Read the model definition and answer for the solid it produces. Units are mm, in the model's axes. Face numbers are marked on the shaded views. Coordinates: 2 decimals unless noted, no trailing zeros. Loops run counter-clockwise (first coordinate to the right, second up) from the corner with the lowest first, then second, coordinate; pieces in that order, holes last. Notation, with made-up numbers: M -37,28 L -19,28 A27 ccw -19,66 Z; hole C -21.75,6.25 d3. An arc over 180 degrees is marked long. One line per item, written item: value. Start each with the question number.
1. The part is cut by section B-B (z = 19). Write down the section's boundary in (x, y).
2. The part is cut by section A-A (x = 18.5). Write down the section's boundary in (y, z).
3. Determine the mould class of the marked faces 1, 2, 3 and 4 for opening direction Z: +Z half, -Z half, draft (parallel to the pull), parting line (faces both ways), or undercut.
4. Consider probe 1 along Y at (x, z) = (3, 30); probe 2 along Z at (x, y) = (27.5, -49.5); probe 3 along Y at (x, z) = (17.25, 27.5). Determine where each line is inside the solid, lowest interval first.
5. Flat-ended cylindrical pins translate along their axes: pin 1 (5 mm diameter, centred on x = 18.5, y = -61.5, fed in from +Z); pin 2 (8 mm diameter, centred on x = 8, y = -47.5, fed in from +Z); pin 3 (12 mm diameter, centred on x = 12, z = 41, fed in from -Y). Find the tip coordinate at first contact, or state that the pin passes through.
6. The part is cut by section C-C (y = -58). Write down the section's boundary in (x, z), then the cut area to 3 significant figures.
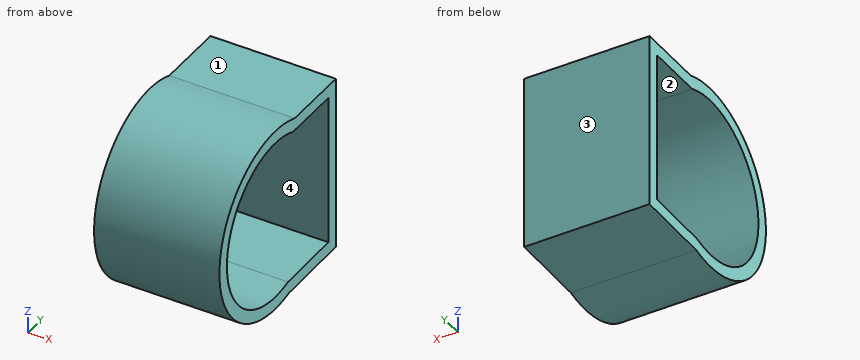
```python
from build123d import *

# Parameters (mm, degrees)
F1_DEPTH = 30
F2_T     = 3


with BuildPart() as f1:
    # F0 (on Right) → F1 (new body)
    with BuildSketch(Plane.YZ):
        with BuildLine():
            ThreePointArc((-50.5638438315, 48.3802992553), (-77.1344876234, 31.6163385121), (-52.6412177761, 11.9412470637))
            Line((-52.6412177761, 11.9412470637), (-36.4591793272, 12.1873354573))
            Line((-36.4591793272, 12.1873354573), (-36.4591793272, 42.854900606))
            Line((-36.4591793272, 42.854900606), (-36.4591793272, 48.3802992553))
            Line((-36.4591793272, 48.3802992553), (-38.9720265736, 48.3802992553))
            Line((-38.9720265736, 48.3802992553), (-50.5638438315, 48.3802992553))
        make_face()
    extrude(amount=F1_DEPTH)

    # F2
    f2_openings = [f1.faces().sort_by_distance(p)[0] for p in [
        (30, -55.280278, 30.40174),
        (0, -55.280278, 30.40174),
    ]]
    offset(amount=F2_T, openings=f2_openings, kind=Kind.INTERSECTION)


solid = f1.part
```
Answer block:
1. outline: M 0,-76.96 L 30,-76.96 L 30,-73.35 L 0,-73.35 Z; M 0,-36.46 L 30,-36.46 L 30,-33.46 L 0,-33.46 Z
2. outline: M -52.22,8.95 L -33.46,9.23 L -33.46,51.38 L -50,51.38 A22.3 ccw long Z; hole M -52.64,11.94 L -36.46,12.19 L -36.46,48.38 L -50.56,48.38 A19.3 ccw long Z
3. face 1: +Z half
3. face 2: undercut
3. face 3: draft
3. face 4: undercut
4. probe 1: y = -80.16 to -77.16, -36.46 to -33.46
4. probe 2: z = 8.99 to 11.99, 48.38 to 51.38
4. probe 3: y = -79.96 to -76.93, -36.46 to -33.46
5. pin 1: stops at z = 52.79
5. pin 2: stops at z = 51.89
5. pin 3: stops at y = -79.71
6. outline: M 0,8.22 L 30,8.22 L 30,11.22 L 0,11.22 Z; M 0,49.82 L 30,49.82 L 30,52.82 L 0,52.82 Z
6. area: 180 mm2
